Input: part model. Units: mm. Frame: model coordinates. Coordinates: 2 decimals unless noted, no trailing zeros. Order: outer loops, then holes, each group sorted by start corner. A loop starts at its lowest first (then second) coordinate and runs counter-clockwise, first axis right, second up. Notation, with made-up numbers: (85, 24) - (126, 24) arc R21 ccw to (126, 46) - close; hole circle Ø5 at (49, 24.25). An arc over 180 degrees is marked (long way). Answer as CSV lines item,"result". Start each with the question number.
Item 1: Draft query along X for faces 1 (the flat face through (175.98, 617, 1568)), 2 (the cylindrical face through (227.647, 613.297, 1568.14)), 3 (the cylindrical face through (236.303, 616.992, 1568.14)), 4 (the flat face through (206, 617, 1572.836)). Return one class per face: +X half, -X half, draft (parallel to the pull), parting line (faces both ways), or undercut.
Item 2: Section D-D (y = 622.5). Output: boundary loops of the cut face in (x, z).
Item 3: Section A-A (x = 230). Output: boundary loops of the cut face in (y, z), and give its area (3 significant figures).
Item 4: First-contact query: pin 1 (1 mm diameter, centred on y = 621.5, z = 1564.5, fed in from +X); pin 2 (2 mm diameter, centred on y = 617.5, z = 1570.5, fed in from +X); pin 3 (1 mm diameter, centred on y = 614.5, z = 1565.5, fed in from +X). Flat tips, straight axial feed; report the tip coordinate or a pass-through.
Item 5: Section B-B (z = 1572). Output: boundary loops of the cut face in (x, y) (3 decimals).
Item 6: Material intervals for line 1 along Y through (x, z) = (227, 1565); line 2 along X through (y, z) = (617.75, 1567); line 3 along X through (y, z) = (618, 1570.5), sorted ascending.
Item 7: Section C-C (y = 614.5). Output: boundary loops of the cut face in (x, z).
from build123d import *

# Parameters (mm, degrees)
BOSS_EXTRUDE1_DEPTH      = 4.7625
BOSS_EXTRUDE1_DEPTH_BACK = 4.7625


with BuildPart() as part:
    # Sketch1 → Boss-Extrude1 (new body, two sides)
    with BuildSketch(Plane.XY.offset(1568.073662845)) as boss_extrude1_sk:
        with BuildLine():
            Line((175.980244033, 626.72659627), (175.980244033, 617.20159627))
            Line((175.980244033, 617.20159627), (175.980244033, 607.67659627))
            Line((175.980244033, 607.67659627), (226.780244033, 607.67659627))
            ThreePointArc((226.780244033, 607.67659627), (236.305244033, 617.20159627), (226.780244033, 626.72659627))
            Line((226.780244033, 626.72659627), (175.980244033, 626.72659627))
        make_face()
        with BuildLine():
            ThreePointArc((230.780244033, 617.20159627), (226.780244033, 613.20159627), (222.780244033, 617.20159627))
            ThreePointArc((222.780244033, 617.20159627), (226.780244033, 621.20159627), (230.780244033, 617.20159627))
        make_face(mode=Mode.SUBTRACT)
    extrude(amount=BOSS_EXTRUDE1_DEPTH)
    extrude(boss_extrude1_sk.sketch, amount=-BOSS_EXTRUDE1_DEPTH_BACK)


solid = part.part
Determined:
1,face 1,"-X half"
1,face 2,"undercut"
1,face 3,"+X half"
1,face 4,"draft"
2,outline,"(175.98, 1563.31) - (234.7, 1563.31) - (234.7, 1572.84) - (175.98, 1572.84) - close"
3,outline,"(608.24, 1563.31) - (614.83, 1563.31) - (614.83, 1572.84) - (608.24, 1572.84) - close; (619.58, 1563.31) - (626.17, 1563.31) - (626.17, 1572.84) - (619.58, 1572.84) - close"
3,area,"126 mm^2"
4,pin 1,"stops at x = 235.52"
4,pin 2,"stops at x = 236.31"
4,pin 3,"stops at x = 236.05"
5,outline,"(175.98, 607.677) - (226.78, 607.677) arc R9.525 ccw to (226.78, 626.727) - (175.98, 626.727) - close; hole circle Ø8 at (226.78, 617.202)"
6,line 1,"y = 607.68 to 613.21, 621.2 to 626.72"
6,line 2,"x = 175.98 to 222.82, 230.74 to 236.29"
6,line 3,"x = 175.98 to 222.86, 230.7 to 236.27"
7,outline,"(175.98, 1563.31) - (223.83, 1563.31) - (223.83, 1572.84) - (175.98, 1572.84) - close; (229.73, 1563.31) - (235.91, 1563.31) - (235.91, 1572.84) - (229.73, 1572.84) - close"
